from build123d import *

# Parameters (mm, degrees)
F0_R     = 25
F0_R_2   = 22.5
F1_DEPTH = 190
F2_W     = 70.4685077071
F2_H     = 92.139782384
F3_DEPTH = 30
F4_R     = 22.5
F5_DEPTH = 100
F6_W     = 21.7724195682
F6_H     = 62.1514879167
F7_DEPTH = 100
F9_DEPTH = 100


with BuildPart() as f1:
    # F0 (on Front) → F1 (new body)
    with BuildSketch(Plane.XZ):
        Circle(F0_R)
        Circle(F0_R_2, mode=Mode.SUBTRACT)
    extrude(amount=F1_DEPTH)

    # F2 (on Right) → F3 (join)
    with BuildSketch(Plane.YZ):
        with Locations((-35.2342538536, 20.8604475483)):
            Rectangle(F2_W, F2_H)
    extrude(amount=F3_DEPTH)

    # F4 (on face) → F5 (cut, symmetric)
    with BuildSketch(Plane.XZ.offset(70.4685077071)):
        Circle(F4_R)
    extrude(amount=F5_DEPTH, both=True, mode=Mode.SUBTRACT)

    # F6 (on Top) → F7 (cut)
    with BuildSketch(Plane.XY):
        with Locations((0.3888274077, -31.0757439584)):
            Rectangle(F6_W, F6_H)
    extrude(amount=F7_DEPTH, mode=Mode.SUBTRACT)

    # F8 (on face) → F9 (cut)
    with BuildSketch(Plane.YZ.offset(30)):
        with BuildLine():
            Line((-27.9086115654, 49), (-67.634855788, 49))
            Line((-67.634855788, 49), (-67.634855788, 38.5))
            Line((-67.634855788, 38.5), (-34.384855788, 38.5))
            ThreePointArc((-34.384855788, 38.5), (-32.6355840211, 44.6683008039), (-27.9086115654, 49))
        make_face()
        with BuildLine():
            ThreePointArc((-17.3611000106, 49), (-22.634855788, 50.25), (-27.9086115654, 49))
            Line((-27.9086115654, 49), (-17.3611000106, 49))
        make_face()
        with BuildLine():
            Line((-17.3611000106, 49), (-27.9086115654, 49))
            ThreePointArc((-27.9086115654, 49), (-32.6355840211, 44.6683008039), (-34.384855788, 38.5))
            Line((-34.384855788, 38.5), (-22.634855788, 38.5))
            Line((-22.634855788, 38.5), (-12.634855788, 38.5))
            Line((-12.634855788, 38.5), (-12.634855788, 44.6694813396))
            ThreePointArc((-12.634855788, 44.6694813396), (-14.696956075, 47.1632700608), (-17.3611000106, 49))
        make_face()
        with BuildLine():
            Line((-34.384855788, 38.5), (-67.634855788, 38.5))
            Line((-67.634855788, 38.5), (-67.634855788, 28))
            Line((-67.634855788, 28), (-27.9086115654, 28))
            ThreePointArc((-27.9086115654, 28), (-32.6355840211, 32.3316991961), (-34.384855788, 38.5))
        make_face()
        with BuildLine():
            Line((-12.634855788, 49), (-17.3611000106, 49))
            ThreePointArc((-17.3611000106, 49), (-14.696956075, 47.1632700608), (-12.634855788, 44.6694813396))
            Line((-12.634855788, 44.6694813396), (-12.634855788, 49))
        make_face()
        with BuildLine():
            Line((-22.634855788, 38.5), (-34.384855788, 38.5))
            ThreePointArc((-34.384855788, 38.5), (-32.6355840211, 32.3316991961), (-27.9086115654, 28))
            Line((-27.9086115654, 28), (-17.3611000106, 28))
            ThreePointArc((-17.3611000106, 28), (-14.696956075, 29.8367299392), (-12.634855788, 32.3305186604))
            Line((-12.634855788, 32.3305186604), (-12.634855788, 38.5))
            Line((-12.634855788, 38.5), (-22.634855788, 38.5))
        make_face()
        with BuildLine():
            ThreePointArc((-10.884855788, 38.5), (-11.3308188984, 41.7064388346), (-12.634855788, 44.6694813396))
            Line((-12.634855788, 44.6694813396), (-12.634855788, 38.5))
            Line((-12.634855788, 38.5), (-10.884855788, 38.5))
        make_face()
        with BuildLine():
            Line((-17.3611000106, 28), (-27.9086115654, 28))
            ThreePointArc((-27.9086115654, 28), (-22.634855788, 26.75), (-17.3611000106, 28))
        make_face()
        with BuildLine():
            Line((-10.884855788, 38.5), (-12.634855788, 38.5))
            Line((-12.634855788, 38.5), (-12.634855788, 32.3305186604))
            ThreePointArc((-12.634855788, 32.3305186604), (-11.3308188984, 35.2935611654), (-10.884855788, 38.5))
        make_face()
        with BuildLine():
            ThreePointArc((-12.634855788, 32.3305186604), (-14.696956075, 29.8367299392), (-17.3611000106, 28))
            Line((-17.3611000106, 28), (-12.634855788, 28))
            Line((-12.634855788, 28), (-12.634855788, 32.3305186604))
        make_face()
    extrude(amount=-F9_DEPTH, mode=Mode.SUBTRACT)


solid = f1.part
CAD build for the part. Positions are in the model's coordinates, mm. A direction names the side the tool comes from. Round coordinates to 2 decimals unless told otherwise and drop trailing zeros. Loops run counter-clockwise (first coordinate to the right, second up) from the corner with the lowest first, then second, coordinate; pieces in that order, holes last.
(1) Cut at D-D (x = 20.5). Give the cut face in (y, z), plus the area to 3 significant figures.
(2) Drop flat-ended pins along their axis: pin 1 (5 mm diameter, centred on x = 17.5, z = 45.5, fed in from -Y); pin 2 (2.5 mm diameter, centred on y = -65.5, z = 37, fed in from -X); pin 3 (8 mm diameter, centred on x = 4, y = -139.5, fed in from +Z); pin 4 (4.5 mm diameter, centred on x = 4.5, z = 22.5, fed in from +Y). Give the stop position or say it passes through.
(3) Wall check: line 1 along Z through (x, y) = (0, -104); line 2 along Y through (x, z) = (25, 46). Give the ranges that are in metal, low to high.
(4) Which spindle directions (+Z, -Z, +X, -X, +Y, -Y) get a long thin tool onto all of the face, cutting with end or side? Do faces 5 (the flat face through (0, -67, 51)), 6 (the flat face through (11.275, -25, 53)), 7 (the flat face through (19, 0, 21)), 8 (the flat face through (21, -12.635, 47)). Say none if no direction does.
(5) Two-plate mould, pull along Z, no slides. Class faces 1 (the flat face through (18, -36, 66.93)), 2 (the flat face through (15, -67.635, 39)), 3 (the flat face through (6, -62.151, 58)), 4 (the cylindrical face through (-24.976, -114.781, 1.099)): +Z half, -Z half, draft (parallel to the pull), parting line (faces both ways), or undercut.
(6) Cut at B-B (y = -48). Give the cut face in (x, z).
(7) Cut at A-A (z = 0). Give the cut face in (x, y).
(8) Cut at C-C (x = 4.5). Give the cut face in (y, z), plus the area to 3 significant figures.
Findings below:
1. outline: (-190, -14.31) - (-70.47, -14.31) - (-70.47, -25.21) - (0, -25.21) - (0, -9.27) - (-190, -9.27) - close; (-190, 9.27) - (0, 9.27) - (0, 66.93) - (-70.47, 66.93) - (-70.47, 14.31) - (-190, 14.31) - close; hole (-67.63, 28) - (-27.91, 28) arc R11.75 ccw to (-17.36, 28) - (-12.63, 28) - (-12.63, 32.33) arc R11.75 ccw to (-12.63, 44.67) - (-12.63, 49) - (-17.36, 49) arc R11.75 ccw to (-27.91, 49) - (-67.63, 49) - close
1. area: 5,200 mm2
2. pin 1: stops at y = -70.47
2. pin 2: passes through
2. pin 3: stops at z = 25
2. pin 4: stops at y = -62.15
3. line 1: z = -25 to -22.5, 22.5 to 25
3. line 2: y = -70.47 to -67.63, -12.63 to 0
4. face 5: +Z, -X, +Y, -Y
4. face 6: +Z, +Y
4. face 7: +Z, -Z, +X, -X, +Y
4. face 8: +X, -X
5. face 1: +Z half
5. face 2: undercut
5. face 3: draft
5. face 4: parting line
6. outline: (-10.5, 19.9) - (-10.5, 22.69) arc R25 ccw to (0, -25) - (0, -25.21) - (30, -25.21) - (30, 28) - (11.28, 28) - (11.28, 19.47) arc R22.5 cw (long way) to start; (11.28, 49) - (30, 49) - (30, 66.93) - (11.28, 66.93) - close
7. outline: (-25, -190) - (-22.5, -190) - (-22.5, 0) - (-25, 0) - close; (22.5, -190) - (25, -190) - (25, -70.47) - (30, -70.47) - (30, 0) - (22.5, 0) - close
8. outline: (-190, -24.59) - (-70.47, -24.59) - (-70.47, -25.21) - (0, -25.21) - (0, -22.05) - (-190, -22.05) - close; (-190, 22.05) - (-62.15, 22.05) - (-62.15, 28) - (-67.63, 28) - (-67.63, 49) - (-62.15, 49) - (-62.15, 66.93) - (-70.47, 66.93) - (-70.47, 24.59) - (-190, 24.59) - close
8. area: 1,090 mm2
